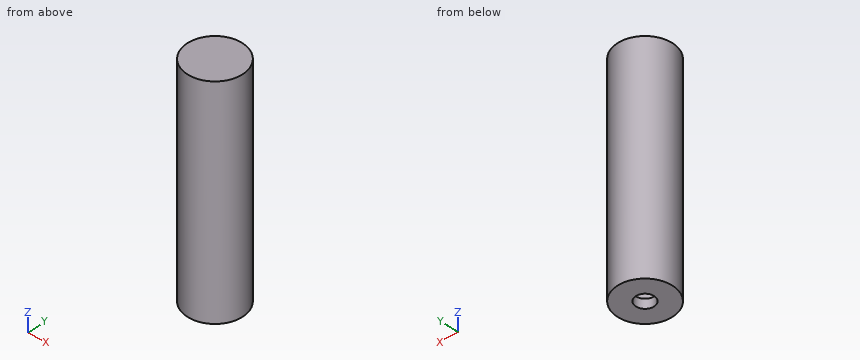
from build123d import *

# Parameters (mm, degrees)
F0_W   = 31.75
F0_H   = 12.7
F0_W_2 = 19.05


with BuildPart() as f1:
    # F0 (on Front) → F1 (revolve)
    with BuildSketch(Plane.XZ):
        with Locations((-15.875, 146.05)):
            Rectangle(F0_W, F0_H)
        Polygon((-31.75, 152.4), (-38.1, 152.4), (-38.1, -152.4), (-31.75, -152.4), (-31.75, -139.7), (-31.75, 139.7), align=None)
        with Locations((-22.225, -146.05)):
            Rectangle(F0_W_2, F0_H)
    revolve(axis=Axis((0, 0, 0), (0, 0, -1)))


solid = f1.part
Verification items for the finished model (mm, model axes). Coordinates: 2 decimals unless noted, no trailing zeros. Loops run counter-clockwise (first coordinate to the right, second up) from the corner with the lowest first, then second, coordinate; pieces in that order, holes last. Notation, with made-up numbers: (-33, 20) -> (9, 20) arc R18 ccw to (9, 54) -> close; hole circle Ø2 at (-7, 1). An arc over 180 degrees is marked (long way). Answer as a JSON object with one key per item and string values. Group by question number.
Item 1: Sectioned sample at C-C on z = -58.5. Record the boundary of the cut face in (x, y), plus the area to 3 significant figures.
Item 2: Depth check by flat-ended pin: pin 1 (3 mm diameter, centred on y = 13, z = 30, fed in from -X); pin 2 (20.5 mm diameter, centred on x = 0, y = 0, fed in from -Z); pin 3 (10 mm diameter, centred on y = 13, z = 104.5, fed in from +X). Enter the tip coordinate at first touch or a pass-through.
Item 3: Sectioned sample at A-A on y = -22. Record the boundary of the cut face in (x, z), plus the area to 3 significant figures.
Item 4: Scan lines: probe 1 along Y at (x, z) = (0, -149); probe 2 along Y at (x, z) = (0, 54); probe 3 along Z at (x, y) = (5, -23). Record each from-to range of solid material in increasing order.
Item 5: Sectioned sample at B-B on x = 24.5. Record the boundary of the cut face in (y, z), plus the area to 3 significant figures.
Item 6: Sectioned sample at D-D on y = 0. Record the boundary of the cut face in (x, z).
Evaluation:
{
 "1": {"outline": "circle Ø76.2 at (0, 0); hole circle Ø63.5 at (0, 0)", "area": "1,390 mm²"},
 "2": {"pin 1": "stops at x = -36.32", "pin 2": "stops at z = 139.7", "pin 3": "stops at x = 37.25"},
 "3": {"outline": "(-31.11, -152.4) -> (31.11, -152.4) -> (31.11, 152.4) -> (-31.11, 152.4) -> close; hole (-22.89, -139.7) -> (22.89, -139.7) -> (22.89, 139.7) -> (-22.89, 139.7) -> close", "area": "6,170 mm²"},
 "4": {"probe 1": "y = -38.1 to -12.7, 12.7 to 38.1", "probe 2": "y = -38.1 to -31.75, 31.75 to 38.1", "probe 3": "z = -152.4 to -139.7, 139.7 to 152.4"},
 "5": {"outline": "(-29.18, -152.4) -> (29.18, -152.4) -> (29.18, 152.4) -> (-29.18, 152.4) -> close; hole (-20.19, -139.7) -> (20.19, -139.7) -> (20.19, 139.7) -> (-20.19, 139.7) -> close", "area": "6,500 mm²"},
 "6": {"outline": "(-38.1, -152.4) -> (-12.7, -152.4) -> (-12.7, -139.7) -> (-31.75, -139.7) -> (-31.75, 139.7) -> (31.75, 139.7) -> (31.75, -139.7) -> (12.7, -139.7) -> (12.7, -152.4) -> (38.1, -152.4) -> (38.1, 152.4) -> (-38.1, 152.4) -> close"}
}
